```python
from build123d import *

# Parameters (mm, degrees)
SKETCH2_W           = 57
SKETCH2_H           = 20
BOSS_EXTRUDE1_DEPTH = 12.5
CUT_EXTRUDE1_DEPTH  = 57


with BuildPart() as part:
    # Sketch2 → Boss-Extrude1 (new body)
    with BuildSketch(Plane(origin=(0, 0, 0), x_dir=(1, 0, 0), z_dir=(0, 1, 0))):
        Rectangle(SKETCH2_W, SKETCH2_H)
    extrude(amount=BOSS_EXTRUDE1_DEPTH)

    # Sketch3 → Cut-Extrude1 (cut)
    with BuildSketch(Plane(origin=(28.5, 0, 0), x_dir=(0, 0, -1), z_dir=(1, 0, 0))):
        with BuildLine():
            Line((-10, 12.5), (-10, 10.22312083))
            ThreePointArc((-10, 10.22312083), (-9.214285714, 11.008835116), (-8.428571429, 10.22312083))
            Line((-8.428571429, 10.22312083), (-8.428571429, 5))
            ThreePointArc((-8.428571429, 5), (-7.678571429, 4.25), (-6.928571429, 5))
            Line((-6.928571429, 5), (-6.928571429, 11.061158869))
            ThreePointArc((-6.928571429, 11.061158869), (-6.142857143, 11.846873154), (-5.357142857, 11.061158869))
            Line((-5.357142857, 11.061158869), (-5.357142857, 5))
            ThreePointArc((-5.357142857, 5), (-4.607142857, 4.25), (-3.857142857, 5))
            Line((-3.857142857, 5), (-3.857142857, 11.552380562))
            ThreePointArc((-3.857142857, 11.552380562), (-3.071428571, 12.338094848), (-2.285714286, 11.552380562))
            Line((-2.285714286, 11.552380562), (-2.285714286, 5))
            ThreePointArc((-2.285714286, 5), (-1.535714286, 4.25), (-0.785714286, 5))
            Line((-0.785714286, 5), (-0.785714286, 11.714285714))
            ThreePointArc((-0.785714286, 11.714285714), (-0.5555839, 12.269869614), (0, 12.5))
            Line((0, 12.5), (-10, 12.5))
        make_face()
    cut_extrude1 = extrude(amount=-CUT_EXTRUDE1_DEPTH, mode=Mode.SUBTRACT)

    # Mirror1: Cut-Extrude1 across plane
    add(cut_extrude1.mirror(Plane.XY), mode=Mode.SUBTRACT)


solid = part.part
```
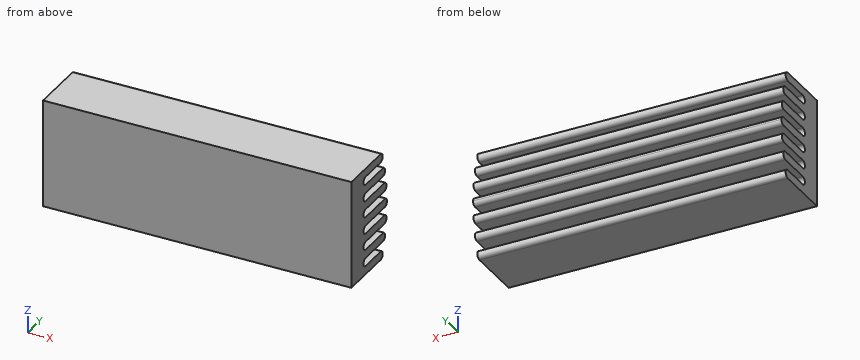
The model under review builds one solid part; all positions refer to its coordinate system, in mm. Round coordinates to 2 decimals unless told otherwise and drop trailing zeros. Order: outer loops, then holes, each group sorted by start corner. A loop starts at its lowest first (then second) coordinate and runs counter-clockwise, first axis right, second up. Notation, with made-up numbers: (76.5, 87.5) -> (115.5, 87.5) arc R31 cw to (115.5, 120.5) -> close; hole circle Ø5 at (-25, -33). An arc over 180 degrees is marked (long way). One line per item, written item: value. Start each with the question number.
Q1. Take a section at C-C (z = 1.5). Write out the cut boundary in (x, y), and give its area (3 significant figures).
Q2. Wall thickness on line 1 (Z direction, x = 5, y = 11.25); line 2 (Y direction, x = 2.5, z = 9.25); line 3 (Z direction, x = 22.5, y = 11.75): over which ranges is each line inside the solid? List them lowest first.
Q3. Take a section at B-B (x = 21). Write out the cut boundary in (y, z).
Q4. Clearance check with flat-ended pins moving along their axes: pin 1 Ø5 at (x, z) = (11.5, -2) entering from -Y; pin 2 Ø6 at (x, z) = (16, -4.5) entering from +Y. State where each tip first meets the part, or that it passes through.
Q5. Take a section at A-A (y = 6). Write out the cut boundary in (x, z), and give its area (3 significant figures).
Reported:
1. outline: (-28.5, 0) -> (28.5, 0) -> (28.5, 4.25) -> (-28.5, 4.25) -> close
1. area: 242 mm2
2. line 1: z = -6.91 to -5.38, -3.86 to -2.29, -0.79 to 0.79, 2.29 to 3.86, 5.38 to 6.91
2. line 2: y = 0 to 11.01
2. line 3: z = -6.52 to -5.76, -3.83 to -2.31, -0.78 to 0.78, 2.31 to 3.83, 5.76 to 6.52
3. outline: (0, -10) -> (10.22, -10) arc R0.79 ccw to (10.22, -8.43) -> (5, -8.43) arc R0.75 cw to (5, -6.93) -> (11.06, -6.93) arc R0.79 ccw to (11.06, -5.36) -> (5, -5.36) arc R0.75 cw to (5, -3.86) -> (11.55, -3.86) arc R0.79 ccw to (11.55, -2.29) -> (5, -2.29) arc R0.75 cw to (5, -0.79) -> (11.71, -0.79) arc R0.79 ccw to (11.71, 0.79) -> (5, 0.79) arc R0.75 cw to (5, 2.29) -> (11.55, 2.29) arc R0.79 ccw to (11.55, 3.86) -> (5, 3.86) arc R0.75 cw to (5, 5.36) -> (11.06, 5.36) arc R0.79 ccw to (11.06, 6.93) -> (5, 6.93) arc R0.75 cw to (5, 8.43) -> (10.22, 8.43) arc R0.79 ccw to (10.22, 10) -> (0, 10) -> close
4. pin 1: stops at y = 0
4. pin 2: stops at y = 12.34
5. outline: (-28.5, -10) -> (28.5, -10) -> (28.5, -8.43) -> (-28.5, -8.43) -> close; (-28.5, -6.93) -> (28.5, -6.93) -> (28.5, -5.36) -> (-28.5, -5.36) -> close; (-28.5, -3.86) -> (28.5, -3.86) -> (28.5, -2.29) -> (-28.5, -2.29) -> close; (-28.5, -0.79) -> (28.5, -0.79) -> (28.5, 0.79) -> (-28.5, 0.79) -> close; (-28.5, 2.29) -> (28.5, 2.29) -> (28.5, 3.86) -> (-28.5, 3.86) -> close; (-28.5, 5.36) -> (28.5, 5.36) -> (28.5, 6.93) -> (-28.5, 6.93) -> close; (-28.5, 8.43) -> (28.5, 8.43) -> (28.5, 10) -> (-28.5, 10) -> close
5. area: 627 mm2
